Here's how the part is built. I have some questions about the finished solid (model axes, mm). Face numbers are marked on the shaded views. A direction names the side the tool comes from. Give positions to 0.01 mm unless a question says otherwise; leave off trailing zeros. Order: outer loops, then holes, each group sorted by start corner. A loop starts at its lowest first (then second) coordinate and runs counter-clockwise, first axis right, second up.
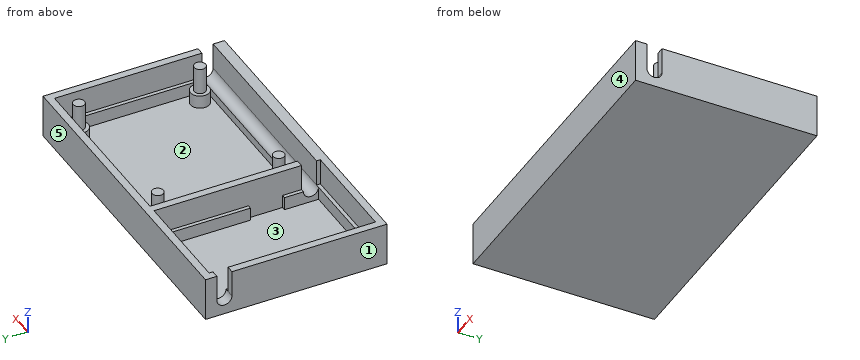
from build123d import *

# Parameters (mm, degrees)
SKETCH005_W     = 82.5
SKETCH005_H     = 48
SKETCH005_W_2   = 28
SKETCH005_H_2   = 44
SKETCH005_W_3   = 48.5
SKETCH005_H_3   = 40.5
PAD003_DEPTH    = 7
SKETCH006_W     = 82.5
SKETCH006_H     = 48
SKETCH006_W_2   = 26
SKETCH006_H_2   = 42
SKETCH006_W_3   = 46.5
SKETCH006_H_3   = 38.5
PAD004_DEPTH    = 3.5
SKETCH007_W     = 82.5
SKETCH007_H     = 48
PAD005_DEPTH    = 1
SKETCH008_R     = 2.5
PAD006_DEPTH    = 3.5
SKETCH009_R     = 1.5
PAD007_DEPTH    = 7
POCKET002_DEPTH = 3.001
POCKET003_DEPTH = 53.501
SKETCH_W        = 1
SKETCH_H        = 9
POCKET_DEPTH    = 3.5


with BuildPart() as part:
    # Sketch005 → Pad003 (new body)
    with BuildSketch(Plane.XY):
        Rectangle(SKETCH005_W, SKETCH005_H)
        with Locations((-25.25, 0)):
            Rectangle(SKETCH005_W_2, SKETCH005_H_2, mode=Mode.SUBTRACT)
        with Locations((15, 1.75)):
            Rectangle(SKETCH005_W_3, SKETCH005_H_3, mode=Mode.SUBTRACT)
    extrude(amount=PAD003_DEPTH)

    # Sketch006 (on Face13 of Pad003) → Pad004 (join)
    with BuildSketch(Plane(origin=(0, 0, 0), x_dir=(1, 0, 0), z_dir=(0, 0, -1))):
        Rectangle(SKETCH006_W, SKETCH006_H)
        with Locations((-25.25, 0)):
            Rectangle(SKETCH006_W_2, SKETCH006_H_2, mode=Mode.SUBTRACT)
        with Locations((15, -1.75)):
            Rectangle(SKETCH006_W_3, SKETCH006_H_3, mode=Mode.SUBTRACT)
    extrude(amount=PAD004_DEPTH)

    # Sketch007 (on Face11 of Pad004) → Pad005 (join)
    with BuildSketch(Plane(origin=(0, 0, -3.5), x_dir=(1, 0, 0), z_dir=(0, 0, -1))):
        Rectangle(SKETCH007_W, SKETCH007_H)
    extrude(amount=PAD005_DEPTH)

    # Sketch008 (on Face22 of Pad005) → Pad006 (join)
    with BuildSketch(Plane.XY.offset(-3.5)):
        with Locations((-5, 17.75)):
            Circle(SKETCH008_R)
        with Locations((35, 17.75)):
            Circle(SKETCH008_R)
        with Locations((35, -14.25)):
            Circle(SKETCH008_R)
        with Locations((-5, -14.25)):
            Circle(SKETCH008_R)
    extrude(amount=PAD006_DEPTH)

    # Sketch009 (on Face34 of Pad006) → Pad007 (join)
    with BuildSketch(Plane.XY):
        with Locations((-5, 17.75)):
            Circle(SKETCH009_R)
        with Locations((35, 17.75)):
            Circle(SKETCH009_R)
        with Locations((35, -14.25)):
            Circle(SKETCH009_R)
        with Locations((-5, -14.25)):
            Circle(SKETCH009_R)
    extrude(amount=PAD007_DEPTH)

    # Sketch010 (on Face21 of Pad007) → Pocket002 (cut, through all)
    with BuildSketch(Plane.YZ.offset(-38.25)):
        with BuildLine():
            Line((21, 0), (21, 7))
            Line((21, 7), (17, 7))
            Line((17, 7), (17, 0))
            ThreePointArc((17, 0), (19, -2), (21, 0))
        make_face()
    extrude(amount=-POCKET002_DEPTH, mode=Mode.SUBTRACT)

    # Sketch011 (on Face25 of Pocket002) → Pocket003 (cut, through all)
    with BuildSketch(Plane(origin=(-12.25, 0, 0), x_dir=(0, -1, 0), z_dir=(-1, 0, 0))):
        with BuildLine():
            Line((21, 0), (21, 7))
            Line((21, 7), (17, 7))
            Line((17, 7), (17, 0))
            ThreePointArc((17, 0), (19, -2), (21, 0))
        make_face()
    extrude(amount=-POCKET003_DEPTH, mode=Mode.SUBTRACT)

    # Sketch (on Face22 of Pocket003) → Pocket (cut)
    with BuildSketch(Plane.XY):
        with Locations((-11.75, -7.5)):
            Rectangle(SKETCH_W, SKETCH_H)
    extrude(amount=-POCKET_DEPTH, mode=Mode.SUBTRACT)


solid = part.part
Q1. I need wall thicknesses on L1, parallel to X at y = -0.5, z = -0.25; L2, parallel to X at y = 8.5, z = 3; L3, parallel to Y at x = -13, z = 4.75. Which ranges of each line are inside material? Lowest first, please.
Filled sheet:
L1: x = -41.25 to -38.25, -12.25 to -8.25, 38.25 to 41.25
L2: x = -41.25 to -39.25, -11.25 to -9.25, 39.25 to 41.25
L3: y = -24 to -22, 22 to 24
Q2. Thinking about a two-plate mould opening in Y: for the marked faces 3, 4 and 5, which applies, released by +Y, released by -Y, zero draft, split by the parting line, or undercut?
Filled sheet:
face 3: undercut
face 4: released by -Y
face 5: released by +Y
Q3. If we section it at B-B on y = 6: List the corners of the cut face in (x, z) for me.
Filled sheet:
outline: (-41.25, -4.5) - (41.25, -4.5) - (41.25, 7) - (39.25, 7) - (39.25, 0) - (38.25, 0) - (38.25, -3.5) - (-8.25, -3.5) - (-8.25, 0) - (-9.25, 0) - (-9.25, 7) - (-11.25, 7) - (-11.25, 0) - (-12.25, 0) - (-12.25, -3.5) - (-38.25, -3.5) - (-38.25, 0) - (-39.25, 0) - (-39.25, 7) - (-41.25, 7) - close
Q4. If we section it at A-A on z = 5.5: List the corners of the cut face in (x, y) for me, plus the area to 3 significant figures.
Filled sheet:
outline: (-41.25, -24) - (41.25, -24) - (41.25, -21) - (-11.25, -21) - (-11.25, -22) - (-39.25, -22) - (-39.25, 17) - (-41.25, 17) - close; (-41.25, 21) - (-39.25, 21) - (-39.25, 22) - (-11.25, 22) - (-11.25, -17) - (-9.25, -17) - (-9.25, 22) - (39.25, 22) - (39.25, -17) - (41.25, -17) - (41.25, 24) - (-41.25, 24) - close; circle Ø3 at (-5, -14.25); circle Ø3 at (-5, 17.75); circle Ø3 at (35, -14.25); circle Ø3 at (35, 17.75)
area: 647 mm2
Q5. For the marked faces 1 and 2, which set-ups out of +Z, -Z, +X, -X, +Y, -Y let a thin tool reach every point of the face, with its end or its side?
Filled sheet:
face 1: +Z, -Z, -X, +Y, -Y
face 2: +Z
Q6. I'm going to push flat-ended pins straight in: P1, Ø2, axis at x = 15.5, y = -5, coming from the +Z side; P2, Ø0.8, axis at x = -11.5, y = -15, coming from the +Z side. Where does each tip first touch, or does it pass through?
Filled sheet:
P1: stops at z = -3.5
P2: stops at z = 7
Q7. If we section it at C-C on x = 35: List the corners of the cut face in (y, z) for me.
Filled sheet:
outline: (-24, -4.5) - (24, -4.5) - (24, 7) - (22, 7) - (22, 0) - (21, 0) - (21, -3.5) - (20.25, -3.5) - (20.25, 0) - (19.25, 0) - (19.25, 7) - (16.25, 7) - (16.25, 0) - (15.25, 0) - (15.25, -3.5) - (-11.75, -3.5) - (-11.75, 0) - (-12.75, 0) - (-12.75, 7) - (-15.75, 7) - (-15.75, 0) - (-16.75, 0) - (-16.75, -3.5) - (-17.5, -3.5) - (-17.5, -1.32) arc R2 cw to (-21, 0) - (-21, 7) - (-24, 7) - close
Q8. If we section it at D-D on x = -13.5: List the corners of the cut face in (y, z) for me, plus the area to 3 significant figures.
Filled sheet:
outline: (-24, -4.5) - (24, -4.5) - (24, 7) - (22, 7) - (22, 0) - (21, 0) - (21, -3.5) - (-21, -3.5) - (-21, 0) - (-22, 0) - (-22, 7) - (-24, 7) - close
area: 97.0 mm2
